The model under review builds one solid part; all positions refer to its coordinate system, in mm. Round coordinates to 2 decimals unless told otherwise and drop trailing zeros. Write each loop counter-clockwise with the first axis right and the second up, starting at its lowest first coordinate (ties: lowest second). Pieces come first, ordered by that corner, then holes. Notation, with made-up numbers: (-4.5, 69) - (37.5, 69) arc R19 ccw to (37.5, 89) - close; hole circle Ø4 at (33.5, 44.25). An arc over 180 degrees is marked (long way). Return JSON: item names as keys, results as strings.
from build123d import *

# Parameters (mm, degrees)
EXTRUDE_1_DEPTH = 20
FILLET_1_R      = 0.5
CHAMFER_1_SIZE  = 0.5


with BuildPart() as part:
    # 草图1 → 凸台-拉伸1 (new body)
    with BuildSketch(Plane.XY):
        with BuildLine():
            Line((-10, -1.5875), (-10, -9.5875))
            Line((-10, -9.5875), (-8.1, -9.5875))
            ThreePointArc((-8.1, -9.5875), (0, -1.4875), (8.1, -9.5875))
            Line((8.1, -9.5875), (10, -9.5875))
            Line((10, -9.5875), (10, -1.5875))
            Line((10, -1.5875), (10, 1.5875))
            Line((10, 1.5875), (-10, 1.5875))
            Line((-10, 1.5875), (-10, -1.5875))
        make_face()
    extrude(amount=EXTRUDE_1_DEPTH)

    # 圆角1
    fillet_1_edges = [part.edges().sort_by_distance(p)[0] for p in [
        (0, -1.4875, 20),
        (0, -1.4875, 0),
    ]]
    fillet(fillet_1_edges, radius=FILLET_1_R)

    # 倒角1
    chamfer_1_edges = [part.edges().sort_by_distance(p)[0] for p in [
        (10, -4, 0),
        (-10, -4, 20),
        (10, -4, 20),
        (-10, -4, 0),
    ]]
    chamfer(chamfer_1_edges, length=CHAMFER_1_SIZE)


solid = part.part
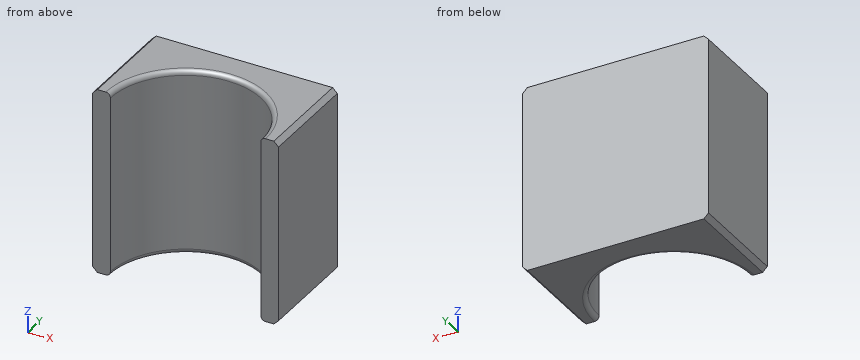
(1) Add section A-A (z = 9.25). Write out the cut boundary in (x, y).
Filled in:
{"outline": "(-10, -9.59) - (-8.1, -9.59) arc R8.1 cw to (8.1, -9.59) - (10, -9.59) - (10, 1.59) - (-10, 1.59) - close"}
(2) Clearance check with flat-ended pins moving along their axes: pin 1 Ø5 at (x, y) = (2, -6.5) entering from -Z; pin 2 Ø6 at (x, z) = (2, 14.5) entering from -Y. State where each tip first meets the part, or that it passes through.
Filled in:
{"pin 1": "passes through", "pin 2": "stops at y = -3.21"}
(3) Add section B-B (x = 0). Write out the cut boundary in (y, z), plus the area to 3 significant figures.
Filled in:
{"outline": "(-1.49, 0.5) arc R0.5 ccw to (-0.99, 0) - (1.59, 0) - (1.59, 20) - (-0.99, 20) arc R0.5 ccw to (-1.49, 19.5) - close", "area": "61.4 mm2"}
(4) Wall thickness on line 1 (X direction, y = -5.75, z = 3.5); line 2 (Y direction, x = 0, z = 12.5); line 3 (X direction, y = -8.75, z = 7.5): over which ranges is each line inside the solid? List them lowest first.
Filled in:
{"line 1": "x = -10 to -7.13, 7.13 to 10", "line 2": "y = -1.49 to 1.59", "line 3": "x = -10 to -8.06, 8.06 to 10"}
